The listing builds one solid part. Answer for the finished solid, in the listing's coordinates (mm). A direction names the side the tool comes from. Coordinates: 2 decimals unless noted, no trailing zeros. Order: outer loops, then holes, each group sorted by start corner. A loop starts at its lowest first (then second) coordinate and runs counter-clockwise, first axis right, second up. Notation, with made-up numbers: (-22, 36.25) -> (-2, 36.25) arc R11 ccw to (-2, 52.25) -> close; hole circle Ø8 at (-4, -39). An arc over 180 degrees is marked (long way). Return JSON: item names as keys, results as strings.
Autodesk Inventor part; units mm, degrees
ref_plane "Work Plane1" through (-6.35, 44.45, 9.525) normal (0, -1, 0) x (1, 0, 0)
ref_plane "YZ Plane" through (0, 0, 0) normal (1, 0, 0) x (0, 1, 0)
ref_plane "XZ Plane" through (0, 0, 0) normal (0, 1, 0) x (-1, 0, 0)
sketch "Sketch1" plane through (0, 0, 0) normal (0, 0, 1) x (1, 0, 0)
  line L0 (-6.35, 0) -> (6.35, 0)
  line L1 (6.35, 0) -> (6.35, 88.9)
  line L2 (6.35, 88.9) -> (-6.35, 88.9)
  line L3 (-6.35, 88.9) -> (-6.35, 0)
  point P0 (0, 0)
  dimension "d6" = 88.9
  dimension "d7" = 12.7
  dimension "d22" = 6.35
extrude "Extrusion3" add sketch "Sketch1" along normal blind 9.525
sketch "Sketch4" plane through (0, 0, 0) normal (0, 0, -1) x (-1, 0, 0)
  line L0 (6.35, 0) -> (-6.35, 0)
  line L1 (-6.35, 0) -> (-6.35, 88.9)
  point P0 (0, 0)
  point P1 (0, 6.35)
  dimension "d13" = 6.35
  dimension "d14" = 6.35
hole "Hole1" at (0, 6.35, 0) direction (0, 0, 1) diameter 6.5278 end through all
sketch "Sketch5" plane through (0, 0, 9.525) normal (0, 0, 1) x (1, 0, 0)
  line L0 (-6.35, 88.9) -> (-6.35, 0)
  line L1 (-6.35, 44.45) -> (6.35, 44.45) construction
  line L2 (6.35, 0) -> (6.35, 88.9)
  point P0 (0, 0)
ref_plane "Work Plane1" through (-6.35, 44.45, 9.525) normal (0, -1, 0) x (1, 0, 0)
mirror "Mirror1" about plane through (-6.35, 44.45, 9.525) normal (0, -1, 0) of "Hole1"
fillet "Fillet1" radius 3.175 4 edges at (-6.35, 88.9, 4.7625) (6.35, 88.9, 4.7625) (6.35, 0, 4.7625) (-6.35, 0, 4.7625)
sketch "Sketch6" plane through (0, 0, 9.525) normal (0, 0, 1) x (1, 0, 0)
  circle A0 centre (0, 6.35) radius 3.2639
  circle A1 centre (0, 6.35) radius 4.7625
  point P0 (0, 0)
  dimension "d25" = 9.525
extrude "Extrusion4" cut sketch "Sketch6" against normal blind 6.35
properties part number "Arm" material "Aluminum 6061"
1. Consider line 1 (Y direction, x = 0, z = 1.8); line 2 (Y direction, x = -0.25, z = 3.5); line 3 (X direction, y = 6.35, z = 1.95). Determine where each line is inside the solid, lowest interval first. Write a range as from..to.
Answer block:
{"line 1": "y = 0..3.09, 9.61..79.29, 85.81..88.9", "line 2": "y = 0..1.59, 11.11..79.3, 85.8..88.9", "line 3": "x = -6.35..-3.26, 3.26..6.35"}
2. The part is cut by section B-B on y = 82.55. Give the vertices of the cut face in (x, z) (3 decimals), and give its area (3 significant figures).
Answer block:
{"outline": "(-6.35, 0) -> (-3.264, 0) -> (-3.264, 9.525) -> (-6.35, 9.525) -> close; (3.264, 0) -> (6.35, 0) -> (6.35, 9.525) -> (3.264, 9.525) -> close", "area": "58.8 mm2"}
3. Each of these flat-tipped pins is pushed along its axis until it touches: pin 1 Ø5 at (x, z) = (-3.5, 7) entering from -Y; pin 2 Ø5.5 at (x, y) = (0, 6.35) entering from -Z. Where does it stop, or does it pass through?
Answer block:
{"pin 1": "stops at y = 0", "pin 2": "passes through"}
4. For faces 4 (the face through (-1.03, 1.7, 6.39)), 5 (the face through (-6.35, 45, 5)), determine the directions among +Z, -Z, +X, -X, +Y, -Y from which every point of the face is accessible in a straight line to the end or side of a thin tool.
Answer block:
{"face 4": "+Z", "face 5": "+Z, -Z, -X, +Y, -Y"}
5. The part is cut by section C-C on z = 8.5. Give the number of separate pieces and of enclosed holes in the cut face, and give its area (3 significant figures).
Answer block:
{"separate pieces": "1", "enclosed holes": "2", "area": "1,020 mm2"}
6. The part is cut by section A-A on x = 0. Give the vertices of the cut face in (y, z) (1 decimal), and give its area (3 significant figures).
Answer block:
{"outline": "(0, 0) -> (3.1, 0) -> (3.1, 3.2) -> (1.6, 3.2) -> (1.6, 9.5) -> (0, 9.5) -> close; (9.6, 0) -> (79.3, 0) -> (79.3, 9.5) -> (11.1, 9.5) -> (11.1, 3.2) -> (9.6, 3.2) -> close; (85.8, 0) -> (88.9, 0) -> (88.9, 9.5) -> (85.8, 9.5) -> close", "area": "703 mm2"}
7. Determine the mould class of faces 1 (the face through (6.35, 44, 5)), 2 (the face through (2.896, 7.856, 1.61)), 3 (the face through (0, 0, 5)) for opening direction Y: pulls with the +Y half, pulls with the -Y half, needs draft (parallel to the pull), parting line crosses it, or undercut.
Answer block:
{"face 1": "needs draft", "face 2": "undercut", "face 3": "pulls with the -Y half"}
